Autodesk Inventor part; units mm, degrees
ref_plane "YZ Plane" through (0, 0, 0) normal (1, 0, 0) x (0, 1, 0)
ref_plane "XZ Plane" through (0, 0, 0) normal (0, 1, 0) x (-1, 0, 0)
ref_plane "XY Plane" through (0, 0, 0) normal (0, 0, 1) x (1, 0, 0)
sketch "Sketch_1" plane through (0, 0, 0) normal (1, 0, 0) x (0, 1, 0)
  line L0 (1, 40) -> (0, 40)
  line L1 (0, 40) -> (0, 0)
  line L2 (0, 0) -> (20, 0)
  line L3 (20, 0) -> (20, 1)
  arc A0 (20, 1) -> (18, 3) centre (18, 1) ccw
  line L4 (18, 3) -> (5, 3)
  arc A1 (3, 5) -> (5, 3) centre (5, 5) ccw
  line L5 (3, 5) -> (3, 38)
  arc A2 (3, 38) -> (1, 40) centre (1, 38) ccw
extrude "Extrusion1" add sketch "Sketch_1" along normal mid plane 18
sketch "Sketch2" plane through (9, 20, 0) normal (0, 0, -1) x (-1, 0, 0)
  point P0 (9, -10)
hole "Hole1" at (0, 10, 0) direction (0, 0, 1) diameter 5.56 depth 3
sketch "Sketch3" plane through (-9, 0, 0) normal (0, -1, 0) x (1, 0, 0)
  point P0 (9, 10)
hole "Hole2" at (0, 0, 10) direction (0, 1, 0) diameter 5.56 depth 3
sketch "Sketch4" plane through (-9, 0, 0) normal (0, -1, 0) x (1, 0, 0)
  point P0 (9, 30)
hole "Hole3" at (0, 0, 30) direction (0, 1, 0) diameter 5.56 depth 3
properties part number "20-4176 Aluminum"
CAD build for the part. Positions are in the model's coordinates, mm. A direction names the side the tool comes from. Give positions to 0.01 mm unless a question says otherwise; leave off trailing zeros. Loops run counter-clockwise (first coordinate to the right, second up) from the corner with the lowest first, then second, coordinate; pieces in that order, holes last. Notation, with made-up numbers: M 43,64 L 82,64 A22 ccw 82,98 Z; hole C -39.5,88 d5. An arc over 180 degrees is marked long. Answer in a Markdown table with one row per item. Add a question column.
Item 1: Drop flat-ended pins along their axis: P1, Ø7, axis at x = 0, z = 30, coming from the +Y side; P2, Ø5, axis at x = 0, y = 10, coming from the -Z side; P3, Ø4, axis at x = 1, y = 13.5, coming from the +Z side. Give the stop position or say it passes through.
Item 2: Tool access for faces 4 (the face through (-0.1, 20, 0.5)), 5 (the face through (0, 13, 3)): list every direction of +Z, -Z, +X, -X, +Y, -Y with a clear straight run to the whole face (end or side of a thin tool).
Item 3: Band-saw the part on A-A on z = 10. Give the cut face in (x, y).
Item 4: Band-saw the part on D-D on x = -6. Give the cut face in (y, z).
Item 5: Band-saw the part on B-B on x = 0. Give the cut face in (y, z).
Item 6: Probe probe 1 along Z at (x, y) = (0, 1.2); probe 2 along X at (y, z) = (1.8, 10); probe 3 along Z at (x, y) = (3.5, 11.5). List the from-to ranges inside material, lowest first.
Item 7: Mould opens along Y. For faces 1 (the face through (-0.13, 2.4, 39.43)), 2 (the face through (-0.1, 0.5, 40)), 3 (the face through (1.06, 12.57, 1.52)) say: +Y half, -Y half, draft (parallel to the pull), parting line (faces both ways), or undercut.
Reply:
| question | item | result |
|---|---|---|
| 1 | P1 | stops at y = 3 |
| 1 | P2 | passes through |
| 1 | P3 | stops at z = 3 |
| 2 | face 4 | +Z, -Z, +X, -X, +Y |
| 2 | face 5 | +Z, +X, -X, +Y |
| 3 | outline | M -9,0 L -2.78,0 L -2.78,3 L -9,3 Z; M 2.78,0 L 9,0 L 9,3 L 2.78,3 Z |
| 4 | outline | M 0,0 L 20,0 L 20,1 A2 ccw 18,3 L 5,3 A2 cw 3,5 L 3,38 A2 ccw 1,40 L 0,40 Z |
| 5 | outline | M 0,0 L 7.22,0 L 7.22,3 L 5,3 A2 cw 3,5 L 3,7.22 L 0,7.22 Z; M 0,12.78 L 3,12.78 L 3,27.22 L 0,27.22 Z; M 0,32.78 L 3,32.78 L 3,38 A2 ccw 1,40 L 0,40 Z; M 12.78,0 L 20,0 L 20,1 A2 ccw 18,3 L 12.78,3 Z |
| 6 | probe 1 | z = 0 to 7.22, 12.78 to 27.22, 32.78 to 39.99 |
| 6 | probe 2 | x = -9 to -2.78, 2.78 to 9 |
| 6 | probe 3 | z = 0 to 3 |
| 7 | face 1 | +Y half |
| 7 | face 2 | draft |
| 7 | face 3 | undercut |
